from build123d import *

# Parameters (mm, degrees)
SKETCH1_W                       = 42
SKETCH1_H                       = 42
BOSS_EXTRUDE2_DEPTH             = 8
SKETCH2_R                       = 11
BOSS_EXTRUDE3_DEPTH             = 2
SKETCH4_W                       = 42
SKETCH4_H                       = 42
BOSS_EXTRUDE5_DEPTH             = 24
SKETCH5_W                       = 42
SKETCH5_H                       = 42
BOSS_EXTRUDE6_DEPTH             = 10
FILLET1_R                       = 4.5
SKETCH7_R                       = 8.75
CUT_EXTRUDE1_DEPTH              = 2
CUT_EXTRUDE2_START              = -2
SKETCH8_R                       = 8.75
CUT_EXTRUDE2_DEPTH              = 2
SKETCH9_R                       = 2.5
BOSS_EXTRUDE9_DEPTH             = 24.5
CHAMFER2_SIZE                   = 0.5
M3X0_5_TAPPED_HOLE1_D           = 2.5
M3X0_5_TAPPED_HOLE1_DEPTH       = 5.75
M3X0_5_TAPPED_HOLE1_CSINK_D     = 3.05
M3X0_5_TAPPED_HOLE1_CSINK_ANGLE = 90
M3X0_5_TAPPED_HOLE1_TIP         = 0.751075774
SKETCH12_W                      = 17
SKETCH12_H                      = 7
BOSS_EXTRUDE10_DEPTH            = 1.5
FILLET2_R                       = 1.5
SKETCH13_W                      = 15
SKETCH13_H                      = 5.6
BOSS_EXTRUDE11_DEPTH            = 4.5
CUT_EXTRUDE3_DEPTH              = 4.5
SKETCH16_R                      = 0.125
BOSS_EXTRUDE12_DEPTH            = 3.5
LPATTERN1_COUNT                 = 6
LPATTERN1_PITCH                 = 2


with BuildPart() as part:
    # Sketch1 → Boss-Extrude2 (new body)
    with BuildSketch(Plane.XY):
        with Locations((-8.615384615, -1.788461538)):
            Rectangle(SKETCH1_W, SKETCH1_H)
    extrude(amount=BOSS_EXTRUDE2_DEPTH)

    # Sketch2 → Boss-Extrude3 (add)
    with BuildSketch(Plane.XY.offset(8)):
        with Locations((-8.615384615, -1.788461538)):
            Circle(SKETCH2_R)
    extrude(amount=BOSS_EXTRUDE3_DEPTH)

    # Sketch4 → Boss-Extrude5 (add)
    with BuildSketch(Plane(origin=(0, 0, 0), x_dir=(-1, 0, 0), z_dir=(0, 0, -1))):
        with Locations((8.615384615, -1.788461538)):
            Rectangle(SKETCH4_W, SKETCH4_H)
    extrude(amount=BOSS_EXTRUDE5_DEPTH)

    # Sketch5 → Boss-Extrude6 (add)
    with BuildSketch(Plane(origin=(0, 0, -24), x_dir=(-1, 0, 0), z_dir=(0, 0, -1))):
        with Locations((8.615384615, -1.788461538)):
            Rectangle(SKETCH5_W, SKETCH5_H)
    extrude(amount=BOSS_EXTRUDE6_DEPTH)

    # Fillet1
    fillet1_edges = [part.edges().sort_by_distance(p)[0] for p in [
        (-29.615384615, 19.211538462, -13),
        (12.384615385, 19.211538462, -13),
        (12.384615385, -22.788461538, -13),
        (-29.615384615, -22.788461538, -13),
    ]]
    fillet(fillet1_edges, radius=FILLET1_R)

    # Sketch7 → Cut-Extrude1 (cut)
    with BuildSketch(Plane(origin=(0, 0, -34), x_dir=(-1, 0, 0), z_dir=(0, 0, -1))):
        with Locations((8.615384615, -1.788461538)):
            Circle(SKETCH7_R)
    extrude(amount=-CUT_EXTRUDE1_DEPTH, mode=Mode.SUBTRACT)

    # Sketch8 → Cut-Extrude2 (cut)
    with BuildSketch(Plane.XY.offset(10).offset(CUT_EXTRUDE2_START)):
        with Locations(Location((-8.615384615, -1.788461538, 0), (0, 0, 180))):
            Circle(SKETCH8_R)
    extrude(amount=CUT_EXTRUDE2_DEPTH, mode=Mode.SUBTRACT)

    # Sketch9 → Boss-Extrude9 (add)
    with BuildSketch(Plane.XY.offset(8)):
        with Locations((-8.615384615, -1.788461538)):
            Circle(SKETCH9_R)
    extrude(amount=BOSS_EXTRUDE9_DEPTH)

    # Chamfer2
    chamfer2_edges = [part.edges().sort_by_distance(p)[0] for p in [
        (-11.115384615, -1.788461538, 32.5),
    ]]
    chamfer(chamfer2_edges, length=CHAMFER2_SIZE)

    # M3x0.5 Tapped Hole1
    with Locations(Plane(origin=(-24.115384615, 13.711538462, 8), x_dir=(1, 0, 0), z_dir=(0, 0, 1))):
        with Locations((0, 0), (31, 0), (31, -31), (0, -31)):
            CounterSinkHole(M3X0_5_TAPPED_HOLE1_D / 2, M3X0_5_TAPPED_HOLE1_CSINK_D / 2, depth=M3X0_5_TAPPED_HOLE1_DEPTH, counter_sink_angle=M3X0_5_TAPPED_HOLE1_CSINK_ANGLE)
            with Locations((0, 0, -(M3X0_5_TAPPED_HOLE1_DEPTH + M3X0_5_TAPPED_HOLE1_TIP / 2))):  # 118° drill point
                Cone(0, M3X0_5_TAPPED_HOLE1_D / 2, M3X0_5_TAPPED_HOLE1_TIP, mode=Mode.SUBTRACT)

    # Sketch12 → Boss-Extrude10 (add)
    with BuildSketch(Plane(origin=(0, 19.211538462, 0), x_dir=(1, 0, 0), z_dir=(0, 1, 0))):
        with Locations((-8.615384615, 27.5)):
            Rectangle(SKETCH12_W, SKETCH12_H)
    extrude(amount=BOSS_EXTRUDE10_DEPTH)

    # Fillet2
    fillet2_edges = [part.edges().sort_by_distance(p)[0] for p in [
        (-8.615384615, 20.711538462, -31),
    ]]
    fillet(fillet2_edges, radius=FILLET2_R - 0.0001)  # a hair under: the kernel refuses the full size

    # Sketch13 → Boss-Extrude11 (add)
    with BuildSketch(Plane(origin=(0, 20.711538462, 0), x_dir=(1, 0, 0), z_dir=(0, 1, 0))):
        with Locations((-8.615384615, 26.8)):
            Rectangle(SKETCH13_W, SKETCH13_H)
    extrude(amount=BOSS_EXTRUDE11_DEPTH)

    # Sketch15 → Cut-Extrude3 (cut)
    with BuildSketch(Plane(origin=(0, 25.211538462, 0), x_dir=(1, 0, 0), z_dir=(0, 1, 0))):
        Polygon((-12.365384615, 24), (-12.365384615, 24.5), (-15.615384615, 24.5), (-15.615384615, 29.1), (-1.615384615, 29.1), (-1.615384615, 24.5), (-4.865384615, 24.5), (-4.865384615, 24), align=None)
    extrude(amount=-CUT_EXTRUDE3_DEPTH, mode=Mode.SUBTRACT)

    # Sketch16 → Boss-Extrude12 (add)
    with BuildSketch(Plane(origin=(0, 20.711538462, 0), x_dir=(1, 0, 0), z_dir=(0, 1, 0))):
        with Locations(Location((-13.615384615, 26.8, 0), (0, 0, 90))):
            Circle(SKETCH16_R)
    boss_extrude12 = extrude(amount=BOSS_EXTRUDE12_DEPTH)

    # LPattern1: Boss-Extrude12 ×6
    with Locations(*[(i * LPATTERN1_PITCH, 0, 0) for i in range(1, LPATTERN1_COUNT)]):
        add(boss_extrude12)


solid = part.part
Can you work these out from the model? Positions are in its coordinate system, mm. A direction names the side the tool comes from. Round coordinates to 2 decimals unless told otherwise and drop trailing zeros. Loops run counter-clockwise (first coordinate to the right, second up) from the corner with the lowest first, then second, coordinate; pieces in that order, holes last. Notation, with made-up numbers: (88, 78.5) - (105, 78.5) arc R25 cw to (105, 112.5) - close; hole circle Ø5 at (80.25, -13). An arc over 180 degrees is marked (long way). Write item = value, one per line. Start each with the question number.
(1) For P1, Ø4, axis at x = -24, z = -18.5, coming from the +Y side; P2, Ø3, axis at y = -2.5, z = 17, coming from the +X side; P3, Ø1.3, axis at y = 22, z = -27, coming from the -X side, each with a flat end and sliding along its axis, tell me the tip position at first contact or that it passes through.
(2) For faces 1 (the face through (-6.5, 0, 8)), 2 (the face through (-9, 23, -29.6)), 3 (the face through (-16.115, 23, -27)), which set-ups out of +Z, -Z, +X, -X, +Y, -Y let a thin tool reach every point of the face, with its end or its side?
(3) If we section it at B-B (x = -20.5): Please give me the cut outline in (y, z).
(4) If I drill on probe 1 along Z at (x, y) = (6.5, 1); probe 2 along Z at (x, y) = (-11, 8); probe 3 along Y at (x, z) = (4, -25), over which ranges is the centre line in solid material (lowest first)? Write a range as [from, to].
(5) If we section it at A-A (z = 3): Please give me the cut outline in (x, y).
(6) If we section it at C-C (z = 28): Please give me the cut outline in (x, y).
(7) If we mould it in two halves opening along Y, with no side actions, what happens to faces 4 (the face through (-1.67, -7.11, -33.01)), 5 (the face through (-15.615, 23, -27)), 6 (the face through (11.101, -21.435, -13.294)), 7 (the face through (-24.015, -17.481, 1.629))? For each: released by +Y, released by -Y, zero draft, split by the parting line, or undercut.
(8) If we section it at D-D (y = 16.5): Please give me the cut outline in (x, z).
Ans:
q1.P1 = 19.21
q1.P2 = -6.12
q1.P3 = -16.12
q2.face_1 = +Z
q2.face_2 = -Z, +X, -X, +Y
q2.face_3 = +Z, -Z, -X, +Y
q3.outline = (-22.79, -34) - (19.21, -34) - (19.21, 8) - (-22.79, 8) - close
q4.probe_1 = [-34, 8]
q4.probe_2 = [-34, 10]
q4.probe_3 = [-22.79, 19.21]
q5.outline = (-29.62, -18.29) arc R4.5 ccw to (-25.12, -22.79) - (7.88, -22.79) arc R4.5 ccw to (12.38, -18.29) - (12.38, 14.71) arc R4.5 ccw to (7.88, 19.21) - (-25.12, 19.21) arc R4.5 ccw to (-29.62, 14.71) - close; hole circle Ø2.5 at (-24.12, -17.29); hole circle Ø2.5 at (-24.12, 13.71); hole circle Ø2.5 at (6.88, -17.29); hole circle Ø2.5 at (6.88, 13.71)
q6.outline = circle Ø5 at (-8.62, -1.79)
q7.face_4 = undercut
q7.face_5 = zero draft
q7.face_6 = released by -Y
q7.face_7 = undercut
q8.outline = (-29.24, -34) - (12.01, -34) - (12.01, 8) - (-29.24, 8) - close
